Geometry check sheet. Reference: the model listing, model coordinates, mm. Coordinates: 2 decimals unless noted, no trailing zeros. Loops run counter-clockwise (first coordinate to the right, second up) from the corner with the lowest first, then second, coordinate; pieces in that order, holes last. Notation, with made-up numbers: (81, 84) - (127, 84) arc R25 ccw to (127, 97) - close; hole circle Ø10 at (46, 34.25). An arc over 180 degrees is marked (long way). One line per item, written item: value.
Autodesk Inventor part; units mm, degrees
ref_plane "YZ Plane" through (0, 0, 0) normal (1, 0, 0) x (0, 1, 0)
ref_plane "XZ Plane" through (0, 0, 0) normal (0, 1, 0) x (-1, 0, 0)
ref_plane "XY Plane" through (0, 0, 0) normal (0, 0, 1) x (1, 0, 0)
sketch "Esquisse1" plane through (0, 0, 0) normal (0, 1, 0) x (-1, 0, 0)
  circle A0 centre (0, 0) radius 25 construction
  line L0 (-25, 0) -> (25, 0) construction
  arc A1 (-75, -80.7775) -> (-75, 80.7775) centre (-25, 0) ccw construction
  arc A2 (75, 80.7775) -> (75, -80.7775) centre (25, 0) ccw construction
  line L1 (0, 25) -> (0, 0) construction
  line L2 (-75, 80.7775) -> (75, 80.7775)
  line L3 (-75, -80.7775) -> (75, -80.7775)
  arc A3 (75, -80.7775) -> (75, 80.7775) centre (25, 0) ccw
  arc A4 (-75, 80.7775) -> (-75, -80.7775) centre (-25, 0) ccw
  dimension "d0" = 50
  dimension "d1" = 190
  dimension "d2" = 150
extrude "Extrusion1" add sketch "Esquisse1" along normal blind 4
sketch "Esquisse4" plane through (0, 0, 0) normal (0, -1, 0) x (1, 0, 0)
  line L0 (-50, 40) -> (50, 40) construction
  line L1 (50, 40) -> (50, -40) construction
  line L2 (50, -40) -> (-50, -40) construction
  line L3 (-50, -40) -> (-50, 40) construction
  circle A0 centre (-50, 40) radius 3
  circle A1 centre (50, 40) radius 3
  circle A2 centre (50, -40) radius 3
  circle A3 centre (-50, -40) radius 3
  line L4 (75, 80.7775) -> (-75, 80.7775)
  point P0 (0, 0)
  dimension "d15" = 80
  dimension "d16" = 100
  dimension "d17" = 50
  dimension "d18" = 40
  dimension "d19" = 6
  dimension "d20" = 6
  dimension "d21" = 6
  dimension "d22" = 6
  dimension "d25" = 40.7775
extrude "Extrusion4" cut sketch "Esquisse4" against normal through all
sketch "Esquisse8" plane through (0, 0, 0) normal (0, -1, 0) x (1, 0, 0)
  line L0 (96.5, 35) -> (96.5, -35)
  line L1 (82, 42) -> (96, 42)
  line L2 (96, 42) -> (96, -42)
  line L3 (96, -42) -> (82, -42)
  line L4 (82, -42) -> (82, 42)
  line L5 (96, 21.5) -> (108.5, 21.5)
  line L6 (108.5, 21.5) -> (108.5, -21.5)
  line L7 (108.5, -21.5) -> (96, -21.5)
  line L8 (96, -21.5) -> (96, 21.5)
  line L9 (82, -14.7) -> (76.3, -14.7)
  line L10 (76.3, -14.7) -> (76.3, 14.7)
  line L11 (76.3, 14.7) -> (82, 14.7)
  line L12 (82, 14.7) -> (82, -14.7)
  line L13 (82, 14.7) -> (72, 14.7)
  line L14 (72, 14.7) -> (72, 24.7)
  line L15 (72, 24.7) -> (82, 24.7)
  line L16 (82, 24.7) -> (82, 14.7)
  line L17 (96, 21.5) -> (110.5, 21.5)
  line L18 (110.5, 21.5) -> (110.5, 35.5)
  line L19 (110.5, 35.5) -> (96, 35.5)
  line L20 (96, 35.5) -> (96, 21.5)
  line L21 (96, 42) -> (82, 42)
  line L22 (82, 42) -> (82, 56)
  line L23 (82, 56) -> (96, 56)
  line L24 (96, 56) -> (96, 42)
  line L25 (72, 24.7) -> (82, 14.7) construction
  line L26 (82, 24.7) -> (72, 14.7) construction
  line L27 (110.5, 21.5) -> (96, 35.5) construction
  line L28 (96, 21.5) -> (110.5, 35.5) construction
  line L29 (82, 56) -> (96, 42) construction
  line L30 (82, 42) -> (96, 56) construction
  circle A0 centre (89, 49) radius 3
  circle A1 centre (77, 19.7) radius 3
  circle A2 centre (103.25, 28.5) radius 3
  arc A3 (75, -80.7775) -> (75, 80.7775) centre (25, 0) ccw
  line L31 (108.5, 21.5) -> (115, 21.5)
  line L32 (115, 21.5) -> (115, -21.5)
  line L33 (115, -21.5) -> (108.5, -21.5)
  line L34 (108.5, -21.5) -> (108.5, 21.5)
  line L35 (0, 0) -> (120, 0)
  dimension "d59" = 84
  dimension "d60" = 14
  dimension "d61" = 29.4
  dimension "d62" = 5.7
  dimension "d63" = 12.5
  dimension "d64" = 43
  dimension "d65" = 42
  dimension "d66" = 14.7
  dimension "d67" = 21.5
  dimension "d68" = 14
  dimension "d69" = 14
  dimension "d70" = 14
  dimension "d71" = 10
  dimension "d72" = 10
  dimension "d73" = 6
  dimension "d74" = 6
  dimension "d75" = 6
  dimension "d78" = 6.5
  dimension "d79" = 5
extrude "Extrusion6" cut sketch "Esquisse8" against normal through all contours A0 | A1 | A2
mirror "Symétrie2" about plane through (0, 0, 0) normal (0, 0, 1) of "Extrusion6"
mirror "Symétrie3" about plane through (0, 0, 0) normal (1, 0, 0) of "Extrusion6", "Symétrie2"
sketch "Esquisse11" plane through (0, 4, 0) normal (0, 1, 0) x (1, 0, 0)
  line L0 (15.75, 19.5) -> (55.75, 19.5)
  line L1 (55.75, 19.5) -> (55.75, -19.5)
  line L2 (55.75, -19.5) -> (15.75, -19.5)
  line L3 (15.75, -19.5) -> (15.75, 19.5)
  line L4 (11.75, 23.5) -> (59.75, 23.5)
  line L5 (59.75, 23.5) -> (59.75, -23.5)
  line L6 (59.75, -23.5) -> (11.75, -23.5)
  line L7 (11.75, -23.5) -> (11.75, 23.5)
  point P0 (0, 0)
  dimension "d103" = 40
  dimension "d104" = 48
  dimension "d105" = 4
  dimension "d106" = 47
  dimension "d107" = 39
  dimension "d108" = 4
  dimension "d109" = 23.5
  dimension "d110" = 11.75
hole "Perçage1" at (15.75, 4, -19.5) at (55.75, 4, -19.5) at (55.75, 4, 19.5) at (15.75, 4, 19.5) direction (0, -1, 0) diameter 4 end through all
mirror "Symétrie7" about plane through (0, 0, 0) normal (1, 0, 0) of "Perçage1"
sketch "Esquisse12" plane through (0, 4, 0) normal (0, 1, 0) x (1, 0, 0)
  arc A0 (75, -80.7775) -> (75, 80.7775) centre (25, 0) ccw
  line L0 (92.8709, 20) -> (117.8709, 20)
  line L1 (117.8709, 20) -> (117.8709, -20)
  line L2 (117.8709, -20) -> (92.8709, -20)
  line L3 (92.8709, -20) -> (92.8709, 20)
  arc A1 (117.8709, 20) -> (117.8709, -20) centre (25, 0) ccw
  arc A2 (117.8709, -20) -> (117.8709, 20) centre (25, 0) ccw
  point P0 (0, 0)
  dimension "d111" = 25
  dimension "d112" = 40
extrude "Extrusion9" cut sketch "Esquisse12" against normal through all contours L1 A0 | L2 L3 L0 L1
mirror "Symétrie8" about plane through (0, 0, 0) normal (1, 0, 0) of "Extrusion9"
sketch "Esquisse14" plane through (0, 0, 0) normal (0, -1, 0) x (1, 0, 0)
  line L0 (75, 80.7775) -> (-75, 80.7775)
  line L1 (-25, 80.7775) -> (25, 80.7775)
  line L2 (25, 80.7775) -> (25, 48.7775)
  line L3 (25, 48.7775) -> (-25, 48.7775)
  line L4 (-25, 48.7775) -> (-25, 80.7775)
  point P0 (0, 0)
  dimension "d131" = 50
  dimension "d132" = 25
  dimension "d133" = 32
extrude "Extrusion11" cut sketch "Esquisse14" against normal through all
mirror "Symétrie10" about plane through (0, 0, 0) normal (0, 0, 1) of "Extrusion11"
equation "\"d20\" = d19"
equation "\"d21\" = d19"
equation "\"d22\" = d19"
equation "\"d65\" = 0.5 * d59"
equation "\"d66\" = 0.5 * d61"
equation "\"d67\" = 0.5 * d64"
equation "\"d68\" = d60"
equation "\"d70\" = d69"
properties part number "base"
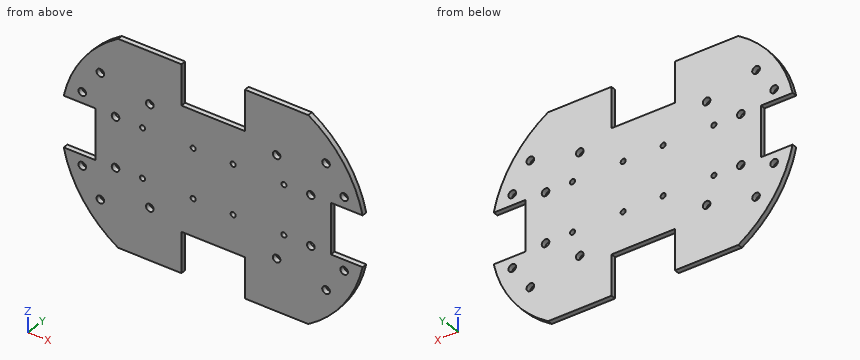
(1) Cross-section at C-C on y = 2.6. State how many separate pieces and enclosed holes the cut face has, and give its area (3 significant figures).
Reply:
separate pieces: 1
enclosed holes: 24
area: 28,600 mm2
(2) Cross-section at B-B on z = -40. Record the cut outline in (x, y).
Reply:
outline: (-111.17, 0) - (-53, 0) - (-53, 4) - (-111.17, 4) - close; (-47, 0) - (47, 0) - (47, 4) - (-47, 4) - close; (53, 0) - (111.17, 0) - (111.17, 4) - (53, 4) - close
(3) Material ranges on probe 1 along Z at (x, y) = (-15.75, 2.2); probe 2 along Z at (x, y) = (55.75, 1.5); probe 3 along X at (y, z) = (2.1, 47), recorded low to high. Write a range as from..to.
Reply:
probe 1: -48.78..-21.5, -17.5..17.5, 21.5..48.78
probe 2: -80.78..-21.5, -17.5..17.5, 21.5..80.78
probe 3: -107.56..-91.24, -86.76..86.76, 91.24..107.56
(4) Go/stop test with flat-tipped pins: pin 1 Ø3.5 at (x, z) = (77, -19.7) entering from +Y; pin 2 Ø2 at (y, z) = (2, 42.5) entering from +X; pin 3 Ø1.5 at (y, z) = (1, -9) entering from +X; pin 4 Ø2 at (x, y) = (-99, 2.5) entering from -Z. Record where each tip stops, or that it passes through.
Reply:
pin 1: through
pin 2: x = 110.46
pin 3: x = 92.87
pin 4: z = -60.79
(5) Cross-section at A-A on x = -50. Record the cut outline in (y, z), and give its area (3 significant figures).
Reply:
outline: (0, -80.78) - (4, -80.78) - (4, -43) - (0, -43) - close; (0, -37) - (4, -37) - (4, 37) - (0, 37) - close; (0, 43) - (4, 43) - (4, 80.78) - (0, 80.78) - close
area: 598 mm2
(6) Cross-section at D-D on x = -103.25. Record the cut outline in (y, z).
Reply:
outline: (0, -53.87) - (4, -53.87) - (4, -31.5) - (0, -31.5) - close; (0, -25.5) - (4, -25.5) - (4, -20) - (0, -20) - close; (0, 20) - (4, 20) - (4, 25.5) - (0, 25.5) - close; (0, 31.5) - (4, 31.5) - (4, 53.87) - (0, 53.87) - close
